For this review, take the finished solid that the model builds, in its own axes (mm). Give positions to 0.01 mm unless a question says otherwise; leave off trailing zeros. Order: outer loops, then holes, each group sorted by start corner. A loop starts at its lowest first (then second) coordinate and runs counter-clockwise, first axis right, second up. Notation, with made-up numbers: (1.25, -20.5) -> (6.25, -20.5) arc R19 cw to (6.25, -1.5) -> close; hole circle Ø6 at (-16, -8). An arc over 180 degrees is marked (long way). Use CSV: the item, a comma, the result in double quotes. Start each with the question number.
```python
from build123d import *

# Parameters (mm, degrees)
RESSALTO_EXTRUS_O1_DEPTH = 2


with BuildPart() as part:
    # Esboço1 → Ressalto-extrusão1 (new body)
    with BuildSketch(Plane.XY):
        with BuildLine():
            Line((-30, 5), (-30, 0))
            Line((-30, 0), (30, 0))
            Line((30, 0), (30, 5))
            Line((30, 5), (40, 5))
            Line((40, 5), (40, 13))
            Line((40, 13), (37.853679508, 13))
            Line((37.853679508, 13), (37.853679508, 10))
            ThreePointArc((37.853679508, 10), (36.820223821, 8.966544314), (35.786768135, 10))
            Line((35.786768135, 10), (35.786768135, 13))
            Line((35.786768135, 13), (30, 13))
            Line((30, 13), (30, 17))
            Line((30, 17), (12, 17))
            Line((12, 17), (12, 10))
            ThreePointArc((12, 10), (11, 9), (10, 10))
            Line((10, 10), (10, 17))
            Line((10, 17), (-10, 17))
            Line((-10, 17), (-10, 10))
            ThreePointArc((-10, 10), (-11, 9), (-12, 10))
            Line((-12, 10), (-12, 17))
            Line((-12, 17), (-30, 17))
            Line((-30, 17), (-30, 13))
            Line((-30, 13), (-35.786768135, 13))
            Line((-35.786768135, 13), (-35.786768135, 10))
            ThreePointArc((-35.786768135, 10), (-36.820223821, 8.966544314), (-37.853679508, 10))
            Line((-37.853679508, 10), (-37.853679508, 13))
            Line((-37.853679508, 13), (-40, 13))
            Line((-40, 13), (-40, 5))
            Line((-40, 5), (-30, 5))
        make_face()
    extrude(amount=RESSALTO_EXTRUS_O1_DEPTH)


solid = part.part
```
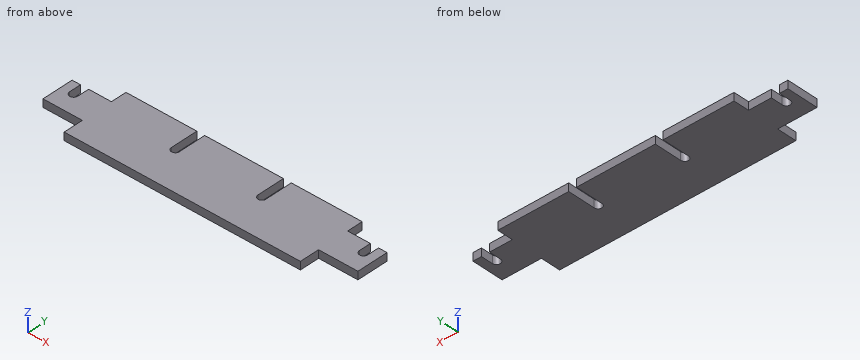
1. To check wall thickness, follow L1, parallel to X at y = 15, z = 0.45; L2, parallel to X at y = 12, z = 0.55; L3, parallel to X at y = 4, z = 0.7. State the ranges of each line that lie inside material, in increasing order. Write a range as [from, to].
2. Consider section C-C (y = 14.25). State the section outline as (x, z) points.
3. Consider section A-A (y = 11). State the section outline as (x, z) points, plus the area to 3 significant figures.
4. Clearance check with flat-ended pins moving along their axes: P1, Ø0.6, axis at y = 15, z = 1, coming from the -X side; P2, Ø0.6, axis at x = 39, z = 0.5, coming from the +Y side. State where each tip first meets the part, or that it passes through.
5. Consider section D-D (x = 11). State the section outline as (y, z) points.
6. Consider section B-B (z = 1.65). State the section outline as (x, y) points.
Answer list:
1,L1,"[-30, -12], [-10, 10], [12, 30]"
1,L2,"[-40, -37.85], [-35.79, -12], [-10, 10], [12, 35.79], [37.85, 40]"
1,L3,"[-30, 30]"
2,outline,"(-30, 0) -> (-12, 0) -> (-12, 2) -> (-30, 2) -> close; (-10, 0) -> (10, 0) -> (10, 2) -> (-10, 2) -> close; (12, 0) -> (30, 0) -> (30, 2) -> (12, 2) -> close"
3,outline,"(-40, 0) -> (-37.85, 0) -> (-37.85, 2) -> (-40, 2) -> close; (-35.79, 0) -> (-12, 0) -> (-12, 2) -> (-35.79, 2) -> close; (-10, 0) -> (10, 0) -> (10, 2) -> (-10, 2) -> close; (12, 0) -> (35.79, 0) -> (35.79, 2) -> (12, 2) -> close; (37.85, 0) -> (40, 0) -> (40, 2) -> (37.85, 2) -> close"
3,area,"144 mm2"
4,P1,"x = -30"
4,P2,"y = 13"
5,outline,"(0, 0) -> (9, 0) -> (9, 2) -> (0, 2) -> close"
6,outline,"(-40, 5) -> (-30, 5) -> (-30, 0) -> (30, 0) -> (30, 5) -> (40, 5) -> (40, 13) -> (37.85, 13) -> (37.85, 10) arc R1.03 cw to (35.79, 10) -> (35.79, 13) -> (30, 13) -> (30, 17) -> (12, 17) -> (12, 10) arc R1 cw to (10, 10) -> (10, 17) -> (-10, 17) -> (-10, 10) arc R1 cw to (-12, 10) -> (-12, 17) -> (-30, 17) -> (-30, 13) -> (-35.79, 13) -> (-35.79, 10) arc R1.03 cw to (-37.85, 10) -> (-37.85, 13) -> (-40, 13) -> close"
